For this review, take the finished solid that the model builds, in its own axes (mm). Give positions to 0.01 mm unless a question says otherwise; leave off trailing zeros. Write each loop counter-clockwise with the first axis right and the second up, starting at its lowest first coordinate (ties: lowest second). Pieces come first, ordered by that corner, then holes. Notation, with made-up numbers: M 41.25,1 L 90.25,1 A23 cw 90.25,24 Z; hole C 51.5,83 d5. An arc over 180 degrees is marked long. One line per item, written item: value. Start each with the question number.
Item 1: To check wall thickness, follow probe 1 along Y at (x, z) = (0, 16.8); probe 2 along X at (y, z) = (5.25, 16.25); probe 3 along Y at (x, z) = (0, 6). State the ranges of each line that lie inside material, in increasing order.
Item 2: Consider section A-A, the plane z = 6. Write out the cut boundary in (x, y).
Item 3: Clearance check with flat-ended pins moving along their axes: pin 1 Ø6 at (x, z) = (9.5, 13) entering from -Y; pin 2 Ø4 at (x, y) = (-2, 3) entering from -Z; pin 3 Ø1.5 at (x, y) = (-7.5, -7.5) entering from +Z. State where each tip first meets the part, or that it passes through.
```python
from build123d import *

# Parameters (mm, degrees)
F3_DEPTH = 2.5
F4_SIZE  = 1
F5_SIZE  = 0.5
F6_SIZE  = 0.25


# Not quite as in the source:
# - a feature names something its author has since deleted; it is built from what else it names


with BuildPart() as f1:
    # F0 (on Front) → F1 (revolve)
    with BuildSketch(Plane.XZ):
        Polygon((7, 15), (7, 0), (8, 0), (8, 5), (13.5, 5), (13.5, 19), (11.5, 19), (11.5, 16), (7.5, 16), (7.5, 18), (0, 18), (0, 15), align=None)
    revolve(axis=Axis((0, 0, 16.5), (0, 0, 1)))

    # F2 (on face) → F3 (join)
    with BuildSketch(Plane.XY.offset(16)):
        with BuildLine():
            Line((0.8279795561, 9.4638496319), (1.0022910416, 11.4562390281))
            ThreePointArc((1.0022910416, 11.4562390281), (0, 11.5), (-1.0022910416, 11.4562390281))
            Line((-1.0022910416, 11.4562390281), (-0.8279795561, 9.4638496319))
            ThreePointArc((-0.8279795561, 9.4638496319), (0, 9.5), (0.8279795561, 9.4638496319))
        make_face()
        with BuildLine():
            ThreePointArc((8.8304981344, 7.3669737816), (8.1575715841, 8.1058019869), (7.4230424297, 8.7834185308))
            Line((7.4230424297, 8.7834185308), (6.1641167123, 7.2830892843))
            ThreePointArc((6.1641167123, 7.2830892843), (6.7751488416, 6.723181496), (7.3350566299, 6.1121493667))
            Line((7.3350566299, 6.1121493667), (8.8304981344, 7.3669737816))
        make_face()
        with BuildLine():
            ThreePointArc((11.5, 0), (11.4899071638, 0.4816984201), (11.4596463708, 0.9625513265))
            Line((11.4596463708, 0.9625513265), (9.5662449685, 0.7969001683))
            ThreePointArc((9.5662449685, 0.7969001683), (9.6023953367, -0.0310793878), (9.5662449685, -0.8590589439))
            Line((9.5662449685, -0.8590589439), (11.4542973626, -1.0242421245))
            ThreePointArc((11.4542973626, -1.0242421245), (11.4885686591, -0.5126306323), (11.5, 0))
        make_face()
        with BuildLine():
            ThreePointArc((7.4117695743, -8.7929330588), (8.141359766, -8.1220847792), (8.810476783, -7.3909064976))
            Line((8.810476783, -7.3909064976), (7.385484621, -6.1951961001))
            ThreePointArc((7.385484621, -6.1951961001), (6.8255768326, -6.8062282293), (6.2145447034, -7.3661360177))
            Line((6.2145447034, -7.3661360177), (7.4117695743, -8.7929330588))
        make_face()
        with BuildLine():
            Line((-0.7566636072, -9.5973243563), (-0.9199020931, -11.4631487881))
            ThreePointArc((-0.9199020931, -11.4631487881), (0.0710446065, -11.4997805485), (1.0614630688, -11.450908093))
            Line((1.0614630688, -11.450908093), (0.899295505, -9.5973243563))
            ThreePointArc((0.899295505, -9.5973243563), (0.0713159489, -9.6334747244), (-0.7566636072, -9.5973243563))
        make_face()
        with BuildLine():
            Line((-7.263740681, -6.2456240912), (-8.7349008301, -7.4800740296))
            ThreePointArc((-8.7349008301, -7.4800740296), (-8.0552507812, -8.2074926044), (-7.3152358724, -8.8734054416))
            Line((-7.3152358724, -8.8734054416), (-6.0928007634, -7.4165640088))
            ThreePointArc((-6.0928007634, -7.4165640088), (-6.7038328927, -6.8566562204), (-7.263740681, -6.2456240912))
        make_face()
        with BuildLine():
            Line((-9.4949290196, 0.7255842194), (-11.464890553, 0.8979335212))
            ThreePointArc((-11.464890553, 0.8979335212), (-11.4995475928, -0.1020056943), (-11.4471576619, -1.1011727676))
            Line((-11.4471576619, -1.1011727676), (-9.4949290196, -0.9303748928))
            ThreePointArc((-9.4949290196, -0.9303748928), (-9.5310793878, -0.1023953367), (-9.4949290196, 0.7255842194))
        make_face()
        with BuildLine():
            ThreePointArc((-11.4471576619, -1.1011727676), (-11.4995475928, -0.1020056943), (-11.464890553, 0.8979335212))
            Line((-11.464890553, 0.8979335212), (-11.4873184158, 0.8998957049))
            ThreePointArc((-11.4873184158, 0.8998957049), (-11.5310793878, -0.1023953367), (-11.4873184158, -1.1046863783))
            Line((-11.4873184158, -1.1046863783), (-11.4471576619, -1.1011727676))
        make_face()
        with BuildLine():
            Line((-6.1432287545, 7.2326612933), (-7.4288039739, 8.7647501795))
            ThreePointArc((-7.4288039739, 8.7647501795), (-8.1684744461, 8.0869670673), (-8.8462575583, 7.347296595))
            Line((-8.8462575583, 7.347296595), (-7.3141686721, 6.0617213757))
            ThreePointArc((-7.3141686721, 6.0617213757), (-6.7542608837, 6.6727535049), (-6.1432287545, 7.2326612933))
        make_face()
    extrude(amount=F3_DEPTH)

    # F4
    f4_edges = [f1.edges().sort_by_distance(p)[0] for p in [
        (-13.5, 0, 19),
        (-7.5, 0, 18),
    ]]
    chamfer(f4_edges, length=F4_SIZE)

    # F5
    f5_edges = [f1.edges().sort_by_distance(p)[0] for p in [
        (-10.471043, -1.015774, 18.5),
        (-10.47991, 0.811759, 18.5),
        (-8.080213, 6.704509, 18.5),
        (-6.786016, 7.998706, 18.5),
        (-0.915135, 10.460044, 18.5),
        (0.915135, 10.460044, 18.5),
        (-6.704018, -8.144985, 18.5),
        (-7.999321, -6.862849, 18.5),
        (0.980379, -10.524116, 18.5),
        (-0.838283, -10.530237, 18.5),
        (8.097981, -6.793051, 18.5),
        (6.813157, -8.079535, 18.5),
        (10.512946, 0.879726, 18.5),
        (10.510271, -0.941651, 18.5),
        (8.082777, 6.739562, 18.5),
        (6.79358, 8.033254, 18.5),
    ]]
    chamfer(f5_edges, length=F5_SIZE)

    # F6
    f6_edges = [f1.edges().sort_by_distance(p)[0] for p in [
        (-13.5, 0, 5),
        (-8, 0, 5),
        (-8, 0, 0),
    ]]
    chamfer(f6_edges, length=F6_SIZE)


solid = f1.part
```
Model answer:
1. probe 1: y = -13.5 to -9.63, -7.5 to 7.5, 9.5 to 13.5
1. probe 2: x = -12.44 to -10.23, -5.36 to 5.36, 10.23 to 12.44
1. probe 3: y = -13.5 to -7, 7 to 13.5
2. outline: C 0,0 d27; hole C 0,0 d14
3. pin 1: stops at y = -11.83
3. pin 2: stops at z = 15
3. pin 3: stops at z = 18.5
